Read the model definition and answer for the solid it produces. Units are mm, in the model's axes. Face numbers are marked on the shaded views. A direction names the side the tool comes from. Coordinates: 2 decimals unless noted, no trailing zeros. Loops run counter-clockwise (first coordinate to the right, second up) from the corner with the lowest first, then second, coordinate; pieces in that order, holes last.
Q1. The mould has two halves that part along Y. Classify the marked faces 1, 2, 3 and 4: pulls with the +Y half, pulls with the -Y half, needs draft (parallel to the pull), parting line crosses it, or undercut.
Q2. Flat-ended cylindrical pins translate along their axes: P1, Ø2, axis at y = 1.5, z = -47.5, coming from the -X side; P2, Ø1, axis at y = 6.5, z = -6, coming from the +X side; P3, Ø1.6, axis at x = 1, z = -43, coming from the +Y side; P4, Ø1.8, axis at x = -1, y = 3.5, coming from the +Z side. Find the tip coordinate at first contact, or state that the pin passes through.
Q3. Straight lines are drawn through the part: line 1 (Y direction, x = 0.25, z = -36); line 2 (Y direction, x = 2, z = -21); line 3 (Y direction, x = 10, z = -31.5). For each, find the intervals that lie inside material, in ascending order.
Q4. Section A-A (x = -1.25) is taken. Give the vertices of the cut face in (y, z), then the cut area to 3 significant figures.
Q5. Which of the six approach directions +Z, -Z, +X, -X, +Y, -Y give full straight-line access (tool end or side, diameter ignored) to the marked faces 5 and 6?
Q6. Section B-B (y = 0.75) is taken. Give the vertices of the cut face in (x, z) (3 decimals), then the cut area to 3 significant figures.
from build123d import *

# Parameters (mm, degrees)
SKETCH1_W             = 70
SKETCH1_H             = 7.5
SKETCH1_W_2           = 1.5
BOSS_EXTRUDE1_DEPTH   = 2
SWEEP1_START          = -73
SWEEP1_DEPTH          = 76
SWEEP1_2_DEPTH        = 3
SWEEP1_3_DEPTH        = 3
SWEEP1_START_2        = -62
SWEEP1_4_DEPTH        = 1.5
SWEEP1_START_3        = -48.875
SWEEP1_5_DEPTH        = 1.5
SWEEP1_START_4        = -35.75
SWEEP1_6_DEPTH        = 1.5
SWEEP1_START_5        = -22.625
SWEEP1_7_DEPTH        = 1.5
SWEEP1_START_6        = -9.5
SWEEP1_8_DEPTH        = 1.5
CUT_EXTRUDE1_DEPTH    = 80
SKETCH4_W             = 1
SKETCH4_H             = 2.284825157
BOSS_EXTRUDE2_DEPTH   = 5
BOSS_EXTRUDE2_2_DEPTH = 5
CUT_EXTRUDE2_DEPTH    = 5
BOSS_EXTRUDE3_DEPTH   = 2.284825157
BOSS_EXTRUDE4_DEPTH   = 2.284825157
FILLET1_R             = 1
FILLET2_R             = 0.2


# Read off the part's stored shape, not the designer's step: Sweep1
with BuildPart() as part:
    # Sketch1 → Boss-Extrude1 (new body)
    # profile 1 of 6: a face of its own
    with BuildSketch(Plane(origin=(0, 0, 0), x_dir=(0, 0, -1), z_dir=(1, 0, 0))):
        Polygon((73, 9.5), (73, 7.5), (73, 0), (73, -1.2), (70, -1.2), (-3, -1.2), (-3, 9.5), (70, 9.5), align=None)
        with Locations((35, 3.75)):
            Rectangle(SKETCH1_W, SKETCH1_H, mode=Mode.SUBTRACT)
    # profile 2 of 6: a face of its own
    with BuildSketch(Plane(origin=(0, 0, 0), x_dir=(0, 0, -1), z_dir=(1, 0, 0))):
        with Locations((8.75, 3.75)):
            Rectangle(SKETCH1_W_2, SKETCH1_H)
    # profile 3 of 6: a face of its own
    with BuildSketch(Plane(origin=(0, 0, 0), x_dir=(0, 0, -1), z_dir=(1, 0, 0))):
        with Locations((21.875, 3.75)):
            Rectangle(SKETCH1_W_2, SKETCH1_H)
    # profile 4 of 6: a face of its own
    with BuildSketch(Plane(origin=(0, 0, 0), x_dir=(0, 0, -1), z_dir=(1, 0, 0))):
        with Locations((35, 3.75)):
            Rectangle(SKETCH1_W_2, SKETCH1_H)
    # profile 5 of 6: a face of its own
    with BuildSketch(Plane(origin=(0, 0, 0), x_dir=(0, 0, -1), z_dir=(1, 0, 0))):
        with Locations((48.125, 3.75)):
            Rectangle(SKETCH1_W_2, SKETCH1_H)
    # profile 6 of 6: a face of its own
    with BuildSketch(Plane(origin=(0, 0, 0), x_dir=(0, 0, -1), z_dir=(1, 0, 0))):
        with Locations((61.25, 3.75)):
            Rectangle(SKETCH1_W_2, SKETCH1_H)
    extrude(amount=BOSS_EXTRUDE1_DEPTH)

    # Sweep1 outline → Sweep1 (add)
    with BuildSketch(Plane.XY.offset(SWEEP1_START)):
        with BuildLine():
            Line((2, 0), (2, -1.2))
            ThreePointArc((2, -1.2), (8.51374729, 1.011119259), (12.335406341, 6.730636217))
            Line((12.335406341, 6.730636217), (11.17629535, 7.041219072))
            ThreePointArc((11.17629535, 7.041219072), (7.783233576, 1.963143267), (2, 0))
        make_face()
        with BuildLine():
            Line((2, 9.5), (2, 7.5))
            ThreePointArc((2, 7.5), (3.217522858, 7.913293319), (3.931851653, 8.98236191))
            Line((3.931851653, 8.98236191), (2, 9.5))
        make_face()
    extrude(amount=SWEEP1_DEPTH)

    # Sweep1 2 outline → Sweep1 2 (add)
    with BuildSketch(Plane.XY.offset(SWEEP1_START)):
        with BuildLine():
            Line((2, 7.5), (2, 0))
            ThreePointArc((2, 0), (7.783233576, 1.963143267), (11.17629535, 7.041219072))
            Line((11.17629535, 7.041219072), (3.931851653, 8.98236191))
            ThreePointArc((3.931851653, 8.98236191), (3.217522858, 7.913293319), (2, 7.5))
        make_face()
    extrude(amount=SWEEP1_2_DEPTH)

    # Sweep1 3 outline → Sweep1 3 (add)
    with BuildSketch(Plane.XY):
        with BuildLine():
            Line((2, 7.5), (2, 0))
            ThreePointArc((2, 0), (7.783233576, 1.963143267), (11.17629535, 7.041219072))
            Line((11.17629535, 7.041219072), (3.931851653, 8.98236191))
            ThreePointArc((3.931851653, 8.98236191), (3.217522858, 7.913293319), (2, 7.5))
        make_face()
    extrude(amount=SWEEP1_3_DEPTH)

    # Sweep1 4 outline → Sweep1 4 (add)
    with BuildSketch(Plane.XY.offset(SWEEP1_START_2)):
        with BuildLine():
            Line((2, 7.5), (2, 0))
            ThreePointArc((2, 0), (7.783233576, 1.963143267), (11.17629535, 7.041219072))
            Line((11.17629535, 7.041219072), (3.931851653, 8.98236191))
            ThreePointArc((3.931851653, 8.98236191), (3.217522858, 7.913293319), (2, 7.5))
        make_face()
    extrude(amount=SWEEP1_4_DEPTH)

    # Sweep1 5 outline → Sweep1 5 (add)
    with BuildSketch(Plane.XY.offset(SWEEP1_START_3)):
        with BuildLine():
            Line((2, 7.5), (2, 0))
            ThreePointArc((2, 0), (7.783233576, 1.963143267), (11.17629535, 7.041219072))
            Line((11.17629535, 7.041219072), (3.931851653, 8.98236191))
            ThreePointArc((3.931851653, 8.98236191), (3.217522858, 7.913293319), (2, 7.5))
        make_face()
    extrude(amount=SWEEP1_5_DEPTH)

    # Sweep1 6 outline → Sweep1 6 (add)
    with BuildSketch(Plane.XY.offset(SWEEP1_START_4)):
        with BuildLine():
            Line((2, 7.5), (2, 0))
            ThreePointArc((2, 0), (7.783233576, 1.963143267), (11.17629535, 7.041219072))
            Line((11.17629535, 7.041219072), (3.931851653, 8.98236191))
            ThreePointArc((3.931851653, 8.98236191), (3.217522858, 7.913293319), (2, 7.5))
        make_face()
    extrude(amount=SWEEP1_6_DEPTH)

    # Sweep1 7 outline → Sweep1 7 (add)
    with BuildSketch(Plane.XY.offset(SWEEP1_START_5)):
        with BuildLine():
            Line((2, 7.5), (2, 0))
            ThreePointArc((2, 0), (7.783233576, 1.963143267), (11.17629535, 7.041219072))
            Line((11.17629535, 7.041219072), (3.931851653, 8.98236191))
            ThreePointArc((3.931851653, 8.98236191), (3.217522858, 7.913293319), (2, 7.5))
        make_face()
    extrude(amount=SWEEP1_7_DEPTH)

    # Sweep1 8 outline → Sweep1 8 (add)
    with BuildSketch(Plane.XY.offset(SWEEP1_START_6)):
        with BuildLine():
            Line((2, 7.5), (2, 0))
            ThreePointArc((2, 0), (7.783233576, 1.963143267), (11.17629535, 7.041219072))
            Line((11.17629535, 7.041219072), (3.931851653, 8.98236191))
            ThreePointArc((3.931851653, 8.98236191), (3.217522858, 7.913293319), (2, 7.5))
        make_face()
    extrude(amount=SWEEP1_8_DEPTH)

    # Sketch3 → Cut-Extrude1 (cut)
    with BuildSketch(Plane.XY.offset(3)):
        with BuildLine():
            add(Edge.make_bspline(
                [(0, 9.5), (1.85008807, 9.446594219), (1.503968772, 9.616267019), (3.992528633, 8.966103562)],
                knots=[0, 0, 0, 0, 1, 1, 1, 1], degree=3))
            Line((3.992528633, 8.966103562), (2, 9.5))
            Line((2, 9.5), (0, 9.5))
        make_face()
    extrude(amount=-CUT_EXTRUDE1_DEPTH, mode=Mode.SUBTRACT)



with BuildPart() as body_2:
    # Sketch4 → Boss-Extrude2 (new body)
    with BuildSketch(Plane.ZY):
        with Locations((-69.5, 3.512617973)):
            Rectangle(SKETCH4_W, SKETCH4_H)
    extrude(amount=BOSS_EXTRUDE2_DEPTH)


with BuildPart() as body_3:
    # Sketch4 → Boss-Extrude2 2 (new body)
    with BuildSketch(Plane.ZY):
        with Locations((-0.5, 3.512617973)):
            Rectangle(SKETCH4_W, SKETCH4_H)
    extrude(amount=BOSS_EXTRUDE2_2_DEPTH)


with BuildPart() as cut_extrude2_tool:
    # Sketch5 → Cut-Extrude2 (new body)
    with BuildSketch(Plane(origin=(0, 4.655030551, 0), x_dir=(1, 0, 0), z_dir=(0, 1, 0))):
        Polygon((-4.341933066, 69), (-5, 69.5), (-5, 69), align=None)
        Polygon((-5, 1), (-5, 0.5), (-4.341933066, 1), align=None)
    extrude(amount=-CUT_EXTRUDE2_DEPTH)


with BuildPart() as body_2_1:
    add(body_2.part)

    # Cut-Extrude2: cut by cut_extrude2_tool
    add(cut_extrude2_tool.part, mode=Mode.SUBTRACT)



with BuildPart() as body_3_1:
    add(body_3.part)

    # Cut-Extrude2: cut by cut_extrude2_tool
    add(cut_extrude2_tool.part, mode=Mode.SUBTRACT)


with BuildPart() as body_2_2:
    add(body_2_1.part)

    add(body_3_1.part)  # Boss-Extrude3 merges body 3
    # Sketch6 → Boss-Extrude3 (add)
    with BuildSketch(Plane(origin=(0, 4.655030551, 0), x_dir=(1, 0, 0), z_dir=(0, 1, 0))):
        Polygon((-3, 70.742293059), (-5, 70), (-3, 70), align=None)
        Polygon((-3, 0), (-5, 0), (-3, -0.742293059), align=None)
    extrude(amount=-BOSS_EXTRUDE3_DEPTH)


with BuildPart() as part_1:
    add(part.part)

    add(body_2_2.part)  # Boss-Extrude4 merges body 2
    # Sketch7 → Boss-Extrude4 (add)
    with BuildSketch(Plane(origin=(0, 4.655030551, 0), x_dir=(1, 0, 0), z_dir=(0, 1, 0))):
        Polygon((0, 69), (2, 69), (5.524751143, 70), (0, 70), align=None)
        Polygon((0, 0), (0, 1), (2, 1), (5.524751143, 0), align=None)
    extrude(amount=-BOSS_EXTRUDE4_DEPTH)

    # Fillet1
    # the kernel refuses this fillet: 1 mm, written as the material it takes off along each edge
    with BuildSketch(Plane(origin=(-4.341933066, 5.497044152, -69), x_dir=(1, 0, 0), z_dir=(0, -1, 0))) as fillet1_piece_1:
        with BuildLine():
            CenterArc((FILLET1_R * 0.336805440666, -FILLET1_R), FILLET1_R, 90, 37.22761065)
            Line((-FILLET1_R * 0.268177449166, -FILLET1_R * 0.203761528805), (-FILLET1_R * 0.280277106962, -FILLET1_R * 0.187836759381))
            Line((-FILLET1_R * 0.280277106962, -FILLET1_R * 0.187836759381), (-FILLET1_R * 0.00673610881331, FILLET1_R * 0.02))
            Line((-FILLET1_R * 0.00673610881331, FILLET1_R * 0.02), (FILLET1_R * 0.336805440666, FILLET1_R * 0.02))
            Line((FILLET1_R * 0.336805440666, FILLET1_R * 0.02), (FILLET1_R * 0.336805440666, 0))
        make_face()
    extrude(amount=3.96885236, mode=Mode.SUBTRACT)
    with BuildSketch(Plane(origin=(-5, 0.687101271, -70), x_dir=(0, 0, 1), z_dir=(0, 1, 0))) as fillet1_piece_2:
        with BuildLine():
            CenterArc((0.703254318, 0.979125979), FILLET1_R, 200.362233207, 57.910439257)
            Line((-0.234257231, 0.631171821), (-0.253007462, 0.624212738))
            Line((-0.253007462, 0.624212738), (-0.018750231, -0.006959083))
            Line((-0.018750231, -0.006959083), (0, -0.02))
            ThreePointArc((0, -0.02), (0.25, -0.02), (0.495934914, -0.01958252))
            Line((0.495934914, -0.01958252), (0.5, 0))
        make_face()
    extrude(amount=5.651033402, mode=Mode.SUBTRACT)
    with BuildSketch(Plane(origin=(-5, 0.687101271, 0), x_dir=(0, 0, -1), z_dir=(0, 1, 0))) as fillet1_piece_3:
        with BuildLine():
            CenterArc((0.703254318, -0.979125979), FILLET1_R, 101.727327536, 57.910439257)
            Line((-0.234257231, -0.631171821), (-0.253007462, -0.624212738))
            Line((-0.253007462, -0.624212738), (-0.018750231, 0.006959083))
            Line((-0.018750231, 0.006959083), (0, 0.02))
            ThreePointArc((0, 0.02), (0.25, 0.02), (0.495934914, 0.01958252))
            Line((0.495934914, 0.01958252), (0.5, 0))
        make_face()
    extrude(amount=5.651033402, mode=Mode.SUBTRACT)
    with BuildSketch(Plane(origin=(-4.341933066, 5.497044152, -1), x_dir=(1, 0, 0), z_dir=(0, -1, 0))) as fillet1_piece_4:
        with BuildLine():
            CenterArc((FILLET1_R * 0.336805440666, FILLET1_R), FILLET1_R, 232.77238935, 37.22761065)
            Line((-FILLET1_R * 0.268177449166, FILLET1_R * 0.203761528805), (-FILLET1_R * 0.280277106962, FILLET1_R * 0.187836759381))
            Line((-FILLET1_R * 0.280277106962, FILLET1_R * 0.187836759381), (-FILLET1_R * 0.00673610881331, -FILLET1_R * 0.02))
            Line((-FILLET1_R * 0.00673610881331, -FILLET1_R * 0.02), (FILLET1_R * 0.336805440666, -FILLET1_R * 0.02))
            Line((FILLET1_R * 0.336805440666, -FILLET1_R * 0.02), (FILLET1_R * 0.336805440666, 0))
        make_face()
    extrude(amount=3.96885236, mode=Mode.SUBTRACT)

    # Fillet2
    fillet2_edges = [part_1.edges().sort_by_distance(p)[0] for p in [
        (-5, 3.512617972, -69.5),
        (-5, 3.512617972, -0.5),
    ]]
    fillet(fillet2_edges, radius=FILLET2_R)


solid = part_1.part
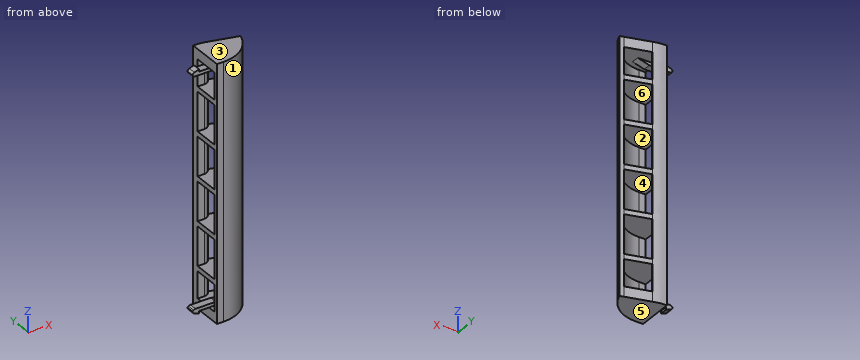
Numbers:
1. face 1: pulls with the -Y half
1. face 2: undercut
1. face 3: needs draft
1. face 4: undercut
2. P1: stops at x = 0
2. P2: stops at x = 12.34
2. P3: stops at y = 9.49
2. P4: stops at z = 0
3. line 1: y = -1.2 to 0, 7.5 to 9.49
3. line 2: y = -1.2 to 0, 7.5 to 9.43
3. line 3: y = 2.39 to 4.38
4. outline: (2.37, -70) - (4.66, -70) - (4.66, -69) - (2.37, -69) - close; (2.37, -1) - (4.66, -1) - (4.66, 0) - (2.37, 0) - close
4. area: 4.57 mm2
5. face 5: -Z, +X, -X, +Y, -Y
5. face 6: none
6. outline: (0, -73) - (8.159, -73) - (8.159, 3) - (0, 3) - (0, 0) - (5.7, 0) - (5.7, -8) - (0, -8) - (0, -9.5) - (5.7, -9.5) - (5.7, -21.125) - (0, -21.125) - (0, -22.625) - (5.7, -22.625) - (5.7, -34.25) - (0, -34.25) - (0, -35.75) - (5.7, -35.75) - (5.7, -47.375) - (0, -47.375) - (0, -48.875) - (5.7, -48.875) - (5.7, -60.5) - (0, -60.5) - (0, -62) - (5.7, -62) - (5.7, -70) - (0, -70) - close
6. area: 264 mm2
